For this review, take the finished solid that the model builds, in its own axes (mm). A direction names the side the tool comes from. Give positions to 0.01 mm unless a question says otherwise; leave off trailing zeros. Loops run counter-clockwise (first coordinate to the right, second up) from the corner with the lowest first, then second, coordinate; pieces in that order, holes last.
```python
from build123d import *

# Parameters (mm, degrees)
SKETCH1_W                    = 514.4008
SKETCH1_H                    = 485.8004
BOSS_EXTRUDE1_DEPTH          = 1.6002
EDGE_FLANGE1_STRIP_W         = 9.6012
EDGE_FLANGE1_STRIP_H         = 1.6002
EDGE_FLANGE1_STRIP_CUT_DEPTH = 485.8004
EDGE_FLANGE1_DEPTH           = 485.8004
EDGE_FLANGE2_STRIP_W         = 9.6012
EDGE_FLANGE2_STRIP_H         = 1.6002
EDGE_FLANGE2_STRIP_CUT_DEPTH = 485.8004
EDGE_FLANGE2_DEPTH           = 485.8004
EDGE_FLANGE4_STRIP_W         = 9.6012
EDGE_FLANGE4_STRIP_H         = 1.6002
EDGE_FLANGE4_STRIP_CUT_DEPTH = 511.2004
EDGE_FLANGE4_DEPTH           = 511.2004
SKETCH18_R                   = 3.2639
CUT_EXTRUDE1_DEPTH           = 573.937935837
SKETCH19_R                   = 3.2639
CUT_EXTRUDE2_DEPTH           = 2.54
SKETCH20_R                   = 3.2639
CUT_EXTRUDE3_DEPTH           = 2.54
SKETCH21_R                   = 26.67
CUT_EXTRUDE4_DEPTH           = 357.936067329


# Sheet-metal steps are written as plain solids
with BuildPart() as part:
    # Sketch1 → Boss-Extrude1 (new body)
    with BuildSketch(Plane(origin=(0, 0, 0), x_dir=(1, 0, 0), z_dir=(0, 1, 0))):
        Rectangle(SKETCH1_W, SKETCH1_H)
    extrude(amount=BOSS_EXTRUDE1_DEPTH)

    # Edge-Flange1 strip (across the edge) → Edge-Flange1 strip cut (cut)
    with BuildSketch(Plane(origin=(-257.2004, 0, 242.9002), x_dir=(1, 0, 0), z_dir=(0, 0, -1))):
        with Locations((-3.2004, -0.8001)):
            Rectangle(EDGE_FLANGE1_STRIP_W, EDGE_FLANGE1_STRIP_H)
    extrude(amount=EDGE_FLANGE1_STRIP_CUT_DEPTH, mode=Mode.SUBTRACT)

    # Edge-Flange1 section (across the edge) → Edge-Flange1 (add)
    with BuildSketch(Plane(origin=(-257.2004, 0, 242.9002), x_dir=(1, 0, 0), z_dir=(0, 0, -1))):
        with BuildLine():
            Line((-1.6002, 1.6002), (-1.6002, 23.7998))
            Line((-1.6002, 23.7998), (0, 23.7998))
            Line((0, 23.7998), (0, 1.6002))
            ThreePointArc((0, 1.6002), (0.468687729, 0.468687729), (1.6002, 0))
            Line((1.6002, 0), (1.6002, -1.6002))
            ThreePointArc((1.6002, -1.6002), (-0.662824543, -0.662824543), (-1.6002, 1.6002))
        make_face()
    extrude(amount=EDGE_FLANGE1_DEPTH)

    # Edge-Flange2 strip (across the edge) → Edge-Flange2 strip cut (cut)
    with BuildSketch(Plane(origin=(257.2004, 0, -242.9002), x_dir=(-1, 0, 0), z_dir=(0, 0, 1))):
        with Locations((-3.2004, -0.8001)):
            Rectangle(EDGE_FLANGE2_STRIP_W, EDGE_FLANGE2_STRIP_H)
    extrude(amount=EDGE_FLANGE2_STRIP_CUT_DEPTH, mode=Mode.SUBTRACT)

    # Edge-Flange2 section (across the edge) → Edge-Flange2 (add)
    with BuildSketch(Plane(origin=(257.2004, 0, -242.9002), x_dir=(-1, 0, 0), z_dir=(0, 0, 1))):
        with BuildLine():
            Line((-1.6002, 1.6002), (-1.6002, 23.7998))
            Line((-1.6002, 23.7998), (0, 23.7998))
            Line((0, 23.7998), (0, 1.6002))
            ThreePointArc((0, 1.6002), (0.468687729, 0.468687729), (1.6002, 0))
            Line((1.6002, 0), (1.6002, -1.6002))
            ThreePointArc((1.6002, -1.6002), (-0.662824543, -0.662824543), (-1.6002, 1.6002))
        make_face()
    extrude(amount=EDGE_FLANGE2_DEPTH)

    # Edge-Flange4 strip (across the edge) → Edge-Flange4 strip cut (cut)
    with BuildSketch(Plane(origin=(-255.6002, 0, -242.9002), x_dir=(0, 0, 1), z_dir=(1, 0, 0))):
        with Locations((-3.2004, -0.8001)):
            Rectangle(EDGE_FLANGE4_STRIP_W, EDGE_FLANGE4_STRIP_H)
    extrude(amount=EDGE_FLANGE4_STRIP_CUT_DEPTH, mode=Mode.SUBTRACT)

    # Edge-Flange4 section (across the edge) → Edge-Flange4 (add)
    with BuildSketch(Plane(origin=(-255.6002, 0, -242.9002), x_dir=(0, 0, 1), z_dir=(1, 0, 0))):
        with BuildLine():
            Line((-1.6002, 1.6002), (-1.6002, 23.7998))
            Line((-1.6002, 23.7998), (0, 23.7998))
            Line((0, 23.7998), (0, 1.6002))
            ThreePointArc((0, 1.6002), (0.468687729, 0.468687729), (1.6002, 0))
            Line((1.6002, 0), (1.6002, -1.6002))
            ThreePointArc((1.6002, -1.6002), (-0.662824543, -0.662824543), (-1.6002, 1.6002))
        make_face()
    extrude(amount=EDGE_FLANGE4_DEPTH)

    # Sketch18 → Cut-Extrude1 (cut, through all)
    with BuildSketch(Plane(origin=(258.8006, 0, 0), x_dir=(0, 0, -1), z_dir=(1, 0, 0))):
        with Locations(Location((-217.5002, -13.6398, 0), (0, 0, 90))):
            Circle(SKETCH18_R)
        with Locations(Location((-109.5502, -13.6398, 0), (0, 0, 90))):
            Circle(SKETCH18_R)
        with Locations(Location((-1.6002, -13.6398, 0), (0, 0, 90))):
            Circle(SKETCH18_R)
        with Locations(Location((106.3498, -13.6398, 0), (0, 0, 90))):
            Circle(SKETCH18_R)
        with Locations(Location((214.2998, -13.6398, 0), (0, 0, 90))):
            Circle(SKETCH18_R)
    extrude(amount=-CUT_EXTRUDE1_DEPTH, mode=Mode.SUBTRACT)

    # Sketch19 → Cut-Extrude2 (cut)
    with BuildSketch(Plane(origin=(0, 0, -244.5004), x_dir=(-1, 0, 0), z_dir=(0, 0, -1))):
        with Locations(Location((-217.5002, -13.6398, 0), (0, 0, 90))):
            Circle(SKETCH19_R)
        with Locations(Location((-109.5502, -13.6398, 0), (0, 0, 90))):
            Circle(SKETCH19_R)
        with Locations(Location((-1.6002, -13.6398, 0), (0, 0, 90))):
            Circle(SKETCH19_R)
        with Locations(Location((106.3498, -13.6398, 0), (0, 0, 90))):
            Circle(SKETCH19_R)
        with Locations(Location((214.2998, -13.6398, 0), (0, 0, 90))):
            Circle(SKETCH19_R)
    extrude(amount=-CUT_EXTRUDE2_DEPTH, mode=Mode.SUBTRACT)

    # Sketch20 → Cut-Extrude3 (cut)
    with BuildSketch(Plane(origin=(0, 1.6002, 0), x_dir=(1, 0, 0), z_dir=(0, 1, 0))):
        with Locations(Location((-217.5002, -223.8502, 0), (0, 0, 270))):
            Circle(SKETCH20_R)
        with Locations(Location((-109.5502, -223.8502, 0), (0, 0, 270))):
            Circle(SKETCH20_R)
        with Locations(Location((-1.6002, -223.8502, 0), (0, 0, 270))):
            Circle(SKETCH20_R)
        with Locations(Location((106.3498, -223.8502, 0), (0, 0, 270))):
            Circle(SKETCH20_R)
        with Locations(Location((214.2998, -223.8502, 0), (0, 0, 270))):
            Circle(SKETCH20_R)
    extrude(amount=-CUT_EXTRUDE3_DEPTH, mode=Mode.SUBTRACT)

    # Sketch21 → Cut-Extrude4 (cut, through all)
    with BuildSketch(Plane(origin=(0, 1.6002, 0), x_dir=(1, 0, 0), z_dir=(0, 1, 0))):
        with Locations(Location((0, -3.175, 0), (0, 0, 270))):
            Circle(SKETCH21_R)
    extrude(amount=-CUT_EXTRUDE4_DEPTH, mode=Mode.SUBTRACT)


solid = part.part
```
Item 1: Clearance check with flat-ended pins moving along their axes: pin 1 Ø4 at (x, z) = (-173.5, 114.5) entering from -Y; pin 2 Ø4 at (y, z) = (-13.64, 217.5) entering from -X; pin 3 Ø1 at (x, y) = (257.5, -6) entering from -Z; pin 4 Ø3 at (x, y) = (-134.5, -14) entering from +Z. State where each tip first meets the part, or that it passes through.
Answer:
pin 1: stops at y = 0
pin 2: passes through
pin 3: stops at z = -242.9
pin 4: stops at z = -242.9
Item 2: Take a section at A-A on z = -149.5. Give the boundary of the cut face in (x, y).
Answer:
outline: (-258.8, -23.8) - (-257.2, -23.8) - (-257.2, -1.6) arc R1.6 cw to (-255.6, 0) - (255.6, 0) arc R1.6 cw to (257.2, -1.6) - (257.2, -23.8) - (258.8, -23.8) - (258.8, -1.6) arc R3.2 ccw to (255.6, 1.6) - (-255.6, 1.6) arc R3.2 ccw to (-258.8, -1.6) - close
Item 3: Tool access review of faces 5 (the flat face through (-1, 1, 242.9)), 6 (the flat face through (-4, -13, -242.9)), 7 (the flat face through (257.2, -13, -3)): name each direction out of +Z, -Z, +X, -X, +Y, -Y from which nothing blocks a thin tool from reaching the whole face with its end or side.
Answer:
face 5: +Z, +X, -X, +Y, -Y
face 6: +Z, -Y
face 7: +Z, -Z, -Y
Item 4: The part is to be moulded in two halves that separate along X. For faces 1 (the flat face through (-258.801, -10, 3)), 2 (the flat face through (258.801, -13, -3)), 3 (the flat face through (-4, -13, -244.5)), 4 (the flat face through (-4, 0, -56)), say which applies: released by +X, released by -X, zero draft, split by the parting line, or undercut.
Answer:
face 1: released by -X
face 2: released by +X
face 3: zero draft
face 4: undercut
Item 5: For L1, parallel to X at y = -11.25, z = -147; L2, parallel to Z at x = -193.5, y = -3.25; L3, parallel to Y at x = 128.5, z = -13.5, list the stretches that pass through material, from the lowest coordinate up.
Answer:
L1: x = -258.8 to -257.2, 257.2 to 258.8
L2: z = -244.5 to -242.9
L3: y = 0 to 1.6
